from build123d import *

# Parameters (mm, degrees)
F0_R     = 4.5
F0_R_2   = 6
F1_DEPTH = 100
F2_R     = 1.5
F3_R     = 0.5
F4_SIZE  = 0.5


with BuildPart() as f1:
    # F0 (on Front) → F1 (new body)
    with BuildSketch(Plane.XZ):
        Polygon((4.117647, -21.029412), (21.617647, -21.029412), (21.617647, -3.529412), (16.617647, -3.529412), (16.617647, -6.029412), (11.617647, -6.029412), (11.617647, 8.970588), (16.617647, 8.970588), (16.617647, 6.470588), (21.617647, 6.470588), (21.617647, 23.970588), (4.117647, 23.970588), (4.117647, 18.970588), (6.617647, 18.970588), (6.617647, 13.970588), (-8.382353, 13.970588), (-8.382353, 18.970588), (-5.882353, 18.970588), (-5.882353, 23.970588), (-23.382353, 23.970588), (-23.382353, 6.470588), (-18.382353, 6.470588), (-18.382353, 8.970588), (-13.382353, 8.970588), (-13.382353, -6.029412), (-18.382353, -6.029412), (-18.382353, -3.529412), (-23.382353, -3.529412), (-23.382353, -21.029412), (-5.882353, -21.029412), (-5.882353, -16.029412), (-8.382353, -16.029412), (-8.382353, -11.029412), (6.617647, -11.029412), (6.617647, -16.029412), (4.117647, -16.029412), align=None)
        with Locations((-15.882353, -13.529412)):
            Circle(F0_R, mode=Mode.SUBTRACT)
        with Locations((14.117647, -13.529412)):
            Circle(F0_R, mode=Mode.SUBTRACT)
        with Locations((-0.882353, 1.470588)):
            Circle(F0_R_2, mode=Mode.SUBTRACT)
        with Locations((-15.882353, 16.470588)):
            Circle(F0_R, mode=Mode.SUBTRACT)
        with Locations((14.117647, 16.470588)):
            Circle(F0_R, mode=Mode.SUBTRACT)
    extrude(amount=F1_DEPTH)

    # F2
    f2_edges = [f1.edges().sort_by_distance(p)[0] for p in [
        (21.617647, -50, 23.970588),
        (21.617647, -50, -21.029412),
        (-23.382353, -50, 23.970588),
        (-23.382353, -50, -21.029412),
    ]]
    fillet(f2_edges, radius=F2_R)

    # F3
    f3_edges = [f1.edges().sort_by_distance(p)[0] for p in [
        (-18.382353, -50, 6.470588),
        (-5.882353, -50, 18.970588),
        (4.117647, -50, 18.970588),
        (16.617647, -50, 6.470588),
        (4.117647, -50, -16.029412),
        (16.617647, -50, -3.529412),
        (-5.882353, -50, -16.029412),
        (-18.382353, -50, -3.529412),
    ]]
    fillet(f3_edges, radius=F3_R)

    # F4
    f4_edges = [f1.edges().sort_by_distance(p)[0] for p in [
        (-5.882353, -50, 23.970588),
        (4.117647, -50, 23.970588),
        (21.617647, -50, 6.470588),
        (21.617647, -50, -3.529412),
        (-5.882353, -50, -21.029412),
        (-23.382353, -50, -3.529412),
        (-23.382353, -50, 6.470588),
        (4.117647, -50, -21.029412),
    ]]
    chamfer(f4_edges, length=F4_SIZE)


solid = f1.part
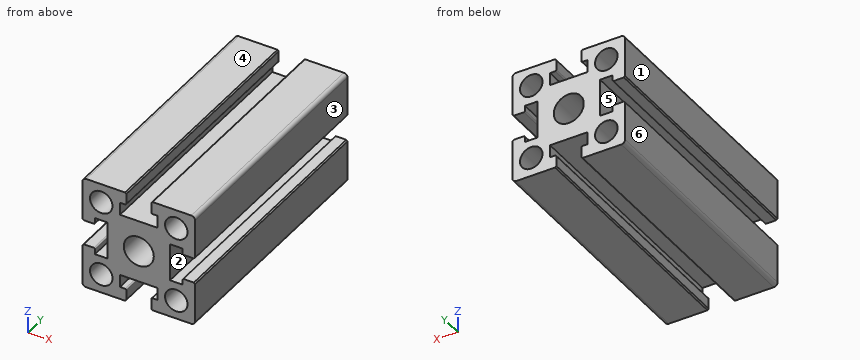
Design review of the part built by this model. Coordinates are the model's own, in mm. Face numbers are marked on the shaded views. A direction names the side the tool comes from. Round coordinates to 2 decimals unless told otherwise and drop trailing zeros. Loops run counter-clockwise (first coordinate to the right, second up) from the corner with the lowest first, then second, coordinate; pieces in that order, holes last. Notation, with made-up numbers: M 52.5,8 L 74.5,8 A13 ccw 74.5,30 Z; hole C -36.75,79 d1. An arc over 180 degrees is marked long. Answer as a JSON object with one key per item and string values.
Item 1: The part is to be moulded in two halves that separate along X. For the marked faces 3, 4, 5 and 6, say which applies: pulls with the +X half, pulls with the -X half, needs draft (parallel to the pull), parting line crosses it, or undercut.
Answer sheet:
{"face 3": "pulls with the +X half", "face 4": "needs draft", "face 5": "undercut", "face 6": "pulls with the -X half"}
Item 2: Clearance check with a flat-ended pin moving along its axis: P1, Ø1.5, axis at x = -0.5, y = -29, coming from the +Z side. State where the tip first meets the part, or that it passes through.
Answer sheet:
{"P1": "stops at z = 13.97"}
Item 3: We need section B-B on x = -2.5. Give the boundary of the cut face in (y, z).
Answer sheet:
{"outline": "M -100,-11.03 L 0,-11.03 L 0,-4.31 L -100,-4.31 Z; M -100,7.25 L 0,7.25 L 0,13.97 L -100,13.97 Z"}
Item 4: We need section C-C on x = 15. Give the boundary of the cut face in (y, z), and give its area (3 significant figures).
Answer sheet:
{"outline": "M -100,-21.03 L 0,-21.03 L 0,-17.94 L -100,-17.94 Z; M -100,-9.12 L 0,-9.12 L 0,-6.03 L -100,-6.03 Z; M -100,8.97 L 0,8.97 L 0,12.06 L -100,12.06 Z; M -100,20.88 L 0,20.88 L 0,23.97 L -100,23.97 Z", "area": "1,230 mm^2"}
Item 5: We need section A-A on z = -15. Give the boundary of the cut face in (x, y).
Answer sheet:
{"outline": "M -23.38,-100 L -20.14,-100 L -20.14,0 L -23.38,0 Z; M -11.63,-100 L -8.38,-100 L -8.38,0 L -11.63,0 Z; M 6.62,-100 L 9.86,-100 L 9.86,0 L 6.62,0 Z; M 18.37,-100 L 21.62,-100 L 21.62,0 L 18.37,0 Z"}
Item 6: Machinability: for the marked faces 1 and 2, which of the approach directions +Z, -Z, +X, -X, +Y, -Y give a long, thin tool a straight path to every point of the face, cutting with its end or side? Answer none if there is none.
Answer sheet:
{"face 1": "+Z, -Z, -X, +Y, -Y", "face 2": "+Y, -Y"}
Item 7: Wall thickness on L1, parallel to Z at x = -16, y = -18.5; L2, parallel to X at y = -74, z = 18; L3, parallel to X at y = -45.5, z = 22: over which ranges is each line inside the solid? List them lowest first. Write a range as from..to.
Answer sheet:
{"L1": "z = -21.03..-18.03, -9.03..-6.03, 8.97..11.97, 20.97..23.97", "L2": "x = -23.38..-20.11, -11.65..-8.38, 6.62..9.89, 18.35..21.62", "L3": "x = -23.38..-5.88, 4.12..21.62"}
Item 8: We need section D-D on y = -33.5. State how many separate pieces and enclosed holes the cut face has, and give its area (3 significant figures).
Answer sheet:
{"separate pieces": "1", "enclosed holes": "5", "area": "1,150 mm^2"}
